Can you work these out from the model? Positions are in its coordinate system, mm. A direction names the side the tool comes from. Coordinates: 2 decimals unless noted, no trailing zeros. Loops run counter-clockwise (first coordinate to the right, second up) from the corner with the lowest first, then second, coordinate; pieces in that order, holes last. Notation, with made-up numbers: (70.5, 82) -> (104.5, 82) arc R14 cw to (104.5, 93) -> close; hole circle Ø5 at (11, 46). An arc over 180 degrees is marked (long way). Use one line per item in the form item = value. Start each with the question number.
(1) I need wall thicknesses on line 1 (Z direction, x = 161, y = 6); line 2 (Y direction, x = 190, z = -8); line 3 (Z direction, x = 55, y = 1.5). Which ranges of each line are inside material? Lowest first, please. Write a range as [from, to].
(2) Imagine slicing it at A-A (z = 0). List the corners of the cut face in (x, y) for me.
(3) I'm going to push flat-ended pins straight in: pin 1 (5 mm diameter, centred on x = 91, z = 4.5, fed in from +Y); pin 2 (3 mm diameter, centred on x = 168, y = 8, fed in from -Z); pin 3 (3 mm diameter, centred on x = 173, z = -0.5, fed in from +Y); pin 4 (2 mm diameter, centred on y = 7, z = 5, fed in from -X). Where does each tip first touch, or does it pass through?
(4) On a 3-axis mill with a long thin cutter (end or side, diameter ignored), from which of +Z, -Z, +X, -X, +Y, -Y can I reach the whole of each face in a straight line? I mean faces 1 (the cylindrical face through (98.61, -9.76, 2.17)), 2 (the flat face through (40, 7, 0)). Say none if no direction works.
(5) Thinking about a two-plate mould opening in X: for faces 3 (the flat face through (200, 0, 0)), 4 (the flat face through (0, 0, 0)), 5 (the flat face through (170, 7, 0)), which applies, released by +X, released by -X, zero draft, split by the parting line, or undercut?
(6) Imagine slicing it at B-B (x = 45). List the corners of the cut face in (y, z) for me, plus the area to 3 significant figures.
(7) Imagine slicing it at C-C (x = 92.5). List the corners of the cut face in (y, z) for me, plus the area to 3 significant figures.
```python
from build123d import *

# Parameters (mm, degrees)
SKETCH_1_R             = 10
EXTRUDE_1_DEPTH        = 200
CUT_EXTRUDE_1_DEPTH    = 3
CHAMFER_1_SIZE         = 1
PATTERN_LINEAR_1_COUNT = 3
PATTERN_LINEAR_1_PITCH = 130
CHAMFER_2_SIZE         = 1


with BuildPart() as part:
    # 草图1 → 凸台-拉伸1 (new body)
    with BuildSketch(Plane(origin=(0, 0, 0), x_dir=(0, 0, -1), z_dir=(1, 0, 0))):
        Circle(SKETCH_1_R)
    extrude(amount=EXTRUDE_1_DEPTH)

    # 草图2 → 切除-拉伸1 (cut)
    with BuildSketch(Plane(origin=(0, 10, 0), x_dir=(1, 0, 0), z_dir=(0, 1, 0))):
        with BuildLine():
            Line((33, 3), (47, 3))
            ThreePointArc((47, 3), (50, 0), (47, -3))
            Line((47, -3), (33, -3))
            ThreePointArc((33, -3), (30, 0), (33, 3))
        make_face()
    cut_extrude_1 = extrude(amount=-CUT_EXTRUDE_1_DEPTH, mode=Mode.SUBTRACT)

    # 倒角1
    chamfer_1_edges = [part.edges().sort_by_distance(p)[0] for p in [
        (0, 0, 10),
    ]]
    chamfer(chamfer_1_edges, length=CHAMFER_1_SIZE)

    # 阵列(线性)1: 切除-拉伸1 ×3
    with Locations(*[(i * PATTERN_LINEAR_1_PITCH, 0, 0) for i in range(1, PATTERN_LINEAR_1_COUNT)]):
        add(cut_extrude_1, mode=Mode.SUBTRACT)

    # 倒角2
    chamfer_2_edges = [part.edges().sort_by_distance(p)[0] for p in [
        (200, 0, 10),
    ]]
    chamfer(chamfer_2_edges, length=CHAMFER_2_SIZE)


solid = part.part
```
Worked out:
q1.line_1 = [-8, 8]
q1.line_2 = [-6, 6]
q1.line_3 = [-9.89, 9.89]
q2.outline = (0, -9) -> (1, -10) -> (199, -10) -> (200, -9) -> (200, 9) -> (199, 10) -> (180, 10) -> (180, 7) -> (160, 7) -> (160, 10) -> (50, 10) -> (50, 7) -> (30, 7) -> (30, 10) -> (1, 10) -> (0, 9) -> close
q3.pin_1 = 9.8
q3.pin_2 = -7.6
q3.pin_3 = 7
q3.pin_4 = 0
q4.face_1 = +X, -X
q4.face_2 = +Y
q5.face_3 = released by +X
q5.face_4 = released by -X
q5.face_5 = undercut
q6.outline = (7, -3) -> (7, 3) -> (9.54, 3) arc R10 ccw (long way) to (9.54, -3) -> close
q6.area = 297 mm2
q7.outline = circle Ø20 at (0, 0)
q7.area = 314 mm2
